```python
from build123d import *

# Parameters (mm, degrees)
F0_W     = 914.4
F0_H     = 25.4
F0_R     = 9.525
F1_DEPTH = 12.7


with BuildPart() as f1:
    # F0 (on Top) → F1 (new body)
    with BuildSketch(Plane.XY):
        with Locations((314.551775, 14.694642)):
            Rectangle(F0_W, F0_H)
        with Locations((-91.848225, 14.694642)):
            Circle(F0_R, mode=Mode.SUBTRACT)
        with Locations((111.351775, 14.694642)):
            Circle(F0_R, mode=Mode.SUBTRACT)
        with Locations((314.551775, 14.694642)):
            Circle(F0_R, mode=Mode.SUBTRACT)
        with Locations((517.751775, 14.694642)):
            Circle(F0_R, mode=Mode.SUBTRACT)
        with Locations((720.951775, 14.694642)):
            Circle(F0_R, mode=Mode.SUBTRACT)
    extrude(amount=F1_DEPTH)


solid = f1.part
```
Model file for the job. Use its own axes, mm. Give positions to 0.01 mm unless a question says otherwise; leave off trailing zeros. Loops run counter-clockwise (first coordinate to the right, second up) from the corner with the lowest first, then second, coordinate; pieces in that order, holes last. Notation, with made-up numbers: (-20, 61) - (-13, 61) arc R19 ccw to (-13, 89) - close; hole circle Ø7 at (65.5, -37). An arc over 180 degrees is marked (long way). One line per item, written item: value. Start each with the question number.
1. Slice it at B-B (z = 3.5). List the corners of the cut face in (x, y) (3 decimals).
2. Slice it at A-A (y = 10.5). List the corners of the cut face in (x, z).
3. Pull direction X, two halves, no side cores. Call faces 1 (the flat face through (308, 6, 0)), 2 (the cylindrical face through (730.037, 17.556, 6.261)): pulls with the +X half, pulls with the -X half, needs draft (parallel to the pull), parting line crosses it, or undercut.
4. Probe L1, parallel to X at y = 14.5, z = 9.5; L2, parallel to X at y = 13.25, z = 12; L3, parallel to Y at x = 320, z = 1.25. List the from-to ranges inside material, lowest first. Write a range as from..to.
Solution:
1. outline: (-142.648, 1.995) - (771.752, 1.995) - (771.752, 27.395) - (-142.648, 27.395) - close; hole circle Ø19.05 at (-91.848, 14.695); hole circle Ø19.05 at (111.352, 14.695); hole circle Ø19.05 at (314.552, 14.695); hole circle Ø19.05 at (517.752, 14.695); hole circle Ø19.05 at (720.952, 14.695)
2. outline: (-142.65, 0) - (-100.4, 0) - (-100.4, 12.7) - (-142.65, 12.7) - close; (-83.3, 0) - (102.8, 0) - (102.8, 12.7) - (-83.3, 12.7) - close; (119.9, 0) - (306, 0) - (306, 12.7) - (119.9, 12.7) - close; (323.1, 0) - (509.2, 0) - (509.2, 12.7) - (323.1, 12.7) - close; (526.3, 0) - (712.4, 0) - (712.4, 12.7) - (526.3, 12.7) - close; (729.5, 0) - (771.75, 0) - (771.75, 12.7) - (729.5, 12.7) - close
3. face 1: needs draft
3. face 2: undercut
4. L1: x = -142.65..-101.37, -82.33..101.83, 120.87..305.03, 324.07..508.23, 527.27..711.43, 730.47..771.75
4. L2: x = -142.65..-101.26, -82.43..101.94, 120.77..305.14, 323.97..508.34, 527.17..711.54, 730.37..771.75
4. L3: y = 1.99..6.88, 22.51..27.39
